Source: three-view drawing plus pictorial views. Frame: mm from the lowest corner of the part. Give positions to 0.01 mm unless a question says otherwise; leave off trailing zeros. Loops run counter-clockwise (first coordinate to the right, second up) from the corner with the lowest first, then second, coordinate; pieces in that order, holes last. Notation, with made-up numbers: M 62.25,50 L 72.25,50 A10 ccw 72.25,64 Z; hole C 11,32.25 d10. An arc over 180 degrees is marked long. One line per item, written item: value. Start each with the question number.
(1) Section D-D on z = 40.5. Output: boundary loops of the cut face in (x, y), plus the area to 3 significant figures.
(2) Section B-B on y = 5. Output: boundary loops of the cut face in (x, z).
(3) Ray query, line 1 along Y through (x, z) = (2.2, 55); line 2 along Z through (x, y) = (1.65, 85); line 3 along Y through (x, z) = (1.5, 56). Return the intervals inside material, ascending. Write a range as from..to.
(4) Section C-C on z = 5. Output: boundary loops of the cut face in (x, y), plus the area to 3 significant figures.
(5) Section A-A on x = 0.7. Output: boundary loops of the cut face in (y, z), plus the area to 3 significant figures.
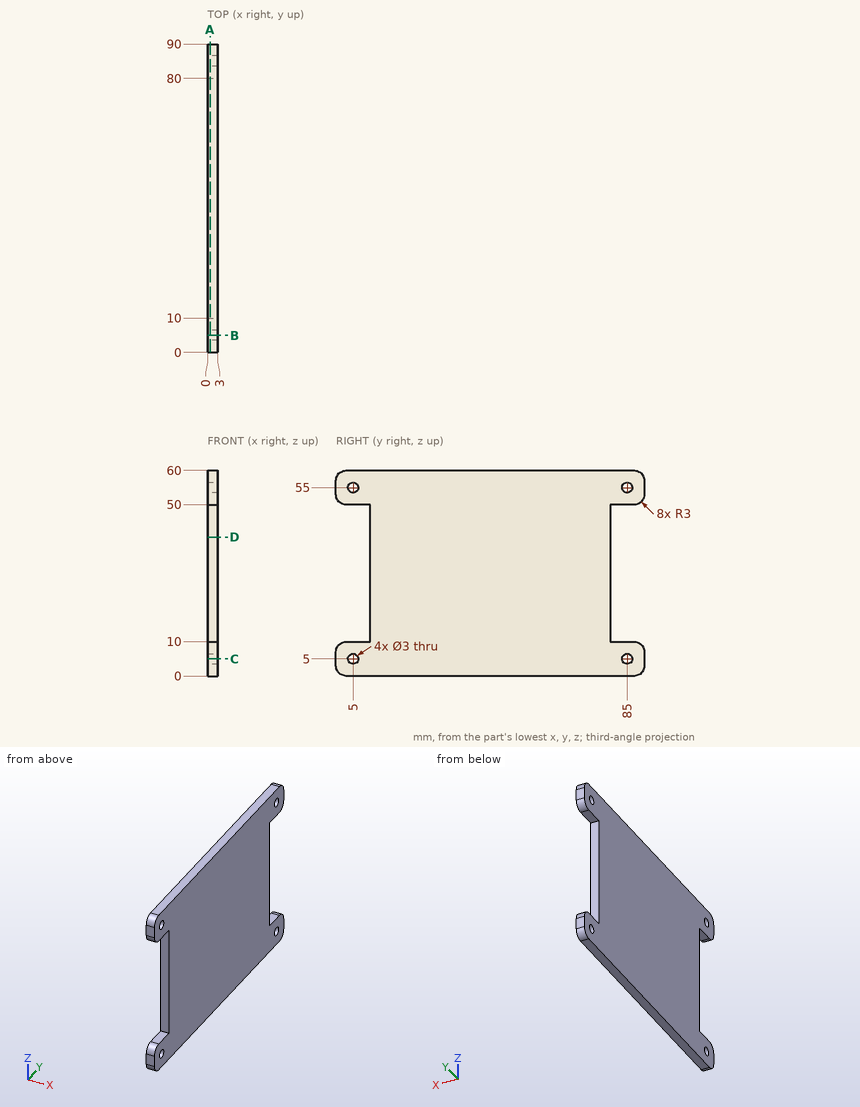
Output values:
1. outline: M 0,10 L 3,10 L 3,80 L 0,80 Z
1. area: 210 mm²
2. outline: M 0,0 L 3,0 L 3,3.5 L 0,3.5 Z; M 0,6.5 L 3,6.5 L 3,10 L 0,10 Z; M 0,50 L 3,50 L 3,53.5 L 0,53.5 Z; M 0,56.5 L 3,56.5 L 3,60 L 0,60 Z
3. line 1: y = 0..3.5, 6.5..83.5, 86.5..90
3. line 2: z = 0..3.5, 6.5..10, 50..53.5, 56.5..60
3. line 3: y = 0..3.88, 6.12..83.88, 86.12..90
4. outline: M 0,0 L 3,0 L 3,3.5 L 0,3.5 Z; M 0,6.5 L 3,6.5 L 3,83.5 L 0,83.5 Z; M 0,86.5 L 3,86.5 L 3,90 L 0,90 Z
4. area: 252 mm²
5. outline: M 0,3 A3 ccw 3,0 L 87,0 A3 ccw 90,3 L 90,7 A3 ccw 87,10 L 80,10 L 80,50 L 87,50 A3 ccw 90,53 L 90,57 A3 ccw 87,60 L 3,60 A3 ccw 0,57 L 0,53 A3 ccw 3,50 L 10,50 L 10,10 L 3,10 A3 ccw 0,7 Z; hole C 5,5 d3; hole C 5,55 d3; hole C 85,5 d3; hole C 85,55 d3
5. area: 4,560 mm²
